```python
from build123d import *

# Parameters (mm, degrees)
SKETCH_1_W          = 15
SKETCH_1_H          = 15
SKETCH_1_W_2        = 12
SKETCH_1_H_2        = 12
EXTRUDE_1_DEPTH     = 220
SKETCH_3_R          = 1.6
CUT_EXTRUDE_2_DEPTH = 221.638278637
SKETCH_4_R          = 2.1
SKETCH_4_R_2        = 1.6
CUT_EXTRUDE_3_DEPTH = 221.638278637


with BuildPart() as part:
    # ｽｹｯﾁ1 → ﾎﾞｽ - 押し出し1 (new body)
    with BuildSketch(Plane(origin=(0, 0, 0), x_dir=(0, 0, -1), z_dir=(1, 0, 0))):
        Rectangle(SKETCH_1_W, SKETCH_1_H)
        Rectangle(SKETCH_1_W_2, SKETCH_1_H_2, mode=Mode.SUBTRACT)
    extrude(amount=EXTRUDE_1_DEPTH)

    # ｽｹｯﾁ3 → ｶｯﾄ - 押し出し2 (cut, through all)
    with BuildSketch(Plane.XY.offset(7.5)):
        with Locations((7.5, 0)):
            Circle(SKETCH_3_R)
        with Locations((212.5, 0)):
            Circle(SKETCH_3_R)
        with Locations((72.5, 0)):
            Circle(SKETCH_3_R)
        with Locations((147.5, 0)):
            Circle(SKETCH_3_R)
    extrude(amount=-CUT_EXTRUDE_2_DEPTH, mode=Mode.SUBTRACT)

    # ｽｹｯﾁ4 → ｶｯﾄ - 押し出し3 (cut, through all)
    with BuildSketch(Plane(origin=(0, 7.5, 0), x_dir=(1, 0, 0), z_dir=(0, 1, 0))):
        with Locations(Location((110, 0, 0), (0, 0, 270))):
            Circle(SKETCH_4_R)
        with Locations(Location((132.5, 0, 0), (0, 0, 270))):
            Circle(SKETCH_4_R_2)
        with Locations(Location((87.5, 0, 0), (0, 0, 270))):
            Circle(SKETCH_4_R_2)
    extrude(amount=-CUT_EXTRUDE_3_DEPTH, mode=Mode.SUBTRACT)


solid = part.part
```
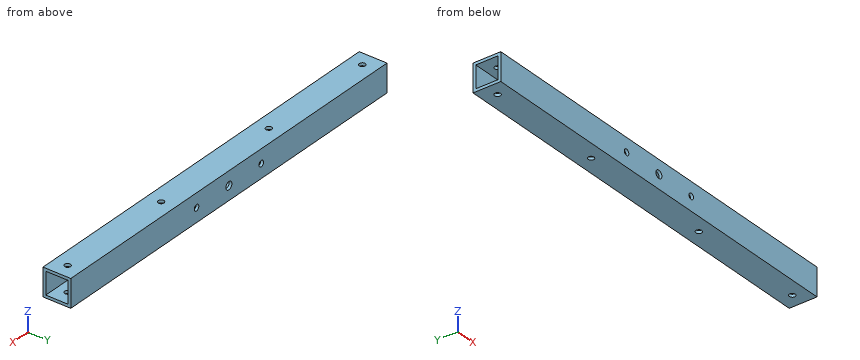
The model under review builds one solid part; all positions refer to its coordinate system, in mm. Round coordinates to 2 decimals unless told otherwise and drop trailing zeros. Order: outer loops, then holes, each group sorted by start corner. A loop starts at its lowest first (then second) coordinate and runs counter-clockwise, first axis right, second up.
(1) Take a section at A-A, the plane y = 3.75. State the section outline as (x, z) points.
Working result:
outline: (0, -7.5) - (220, -7.5) - (220, -6) - (0, -6) - close; (0, 6) - (220, 6) - (220, 7.5) - (0, 7.5) - close
(2) Wall thickness on L1, parallel to Y at x = 17, z = -2.5; L2, parallel to Y at x = 147.5, z = 7.25: over which ranges is each line inside the solid? List them lowest first.
Working result:
L1: y = -7.5 to -6, 6 to 7.5
L2: y = -7.5 to -1.6, 1.6 to 7.5
(3) Take a section at B-B, the plane x = 169.5. State the section outline as (y, z) points.
Working result:
outline: (-7.5, -7.5) - (7.5, -7.5) - (7.5, 7.5) - (-7.5, 7.5) - close; hole (-6, -6) - (6, -6) - (6, 6) - (-6, 6) - close
